The listing builds one solid part. Answer for the finished solid, in the listing's coordinates (mm). A direction names the side the tool comes from. Coordinates: 2 decimals unless noted, no trailing zeros. Order: outer loops, then holes, each group sorted by start corner. A loop starts at its lowest first (then second) coordinate and runs counter-clockwise, first axis right, second up. Notation, with made-up numbers: (20.25, 65.5) - (33.25, 65.5) arc R18 cw to (33.25, 78.5) - close; hole circle Ø7 at (-17.75, 75.25). An arc over 180 degrees is marked (long way). Use one line per item in the form item = value. Start each with the question number.
Item 1: Consider line 1 along Z through (x, y) = (6, -16.25); line 2 along Y through (x, z) = (9.25, 48.75); line 3 along X through (y, z) = (-17.5, 45.25). Determine where each line is inside the solid, lowest interval first. Write a range as [from, to].
Item 2: Section D-D, the plane x = 11.5 is taken. Write down the section's boundary in (y, z), and give its area (3 significant figures).
Item 3: A tool of negligible diameter and unlimited length cuts with its end or side. For faces 1 (the flat face through (10, -20, 46)), 2 (the flat face through (8, -15, 42.675)), from which of +Z, -Z, +X, -X, +Y, -Y can it reach the whole face along a straight path? Write none if from no direction.
Item 4: Section B-B, the plane x = 12.5 is taken. Write down the section's boundary in (y, z).
Item 5: Section A-A, the plane y = -3 is taken. Write down the section's boundary in (x, z).
Item 6: This flat-tipped pin is pushed along its axis until it touches: pin 1 Ø2 at (y, z) = (-16, 48) entering from -X. Where does it stop, or does it pass through?
Item 7: Section C-C, the plane z = 43.75 is taken. Write down the section's boundary in (x, y), and give its area (3 significant figures).
Item 8: The mould has two halves that part along Z. Classify faces 3 (the cylindrical face through (9.897, -3.57, 47.986)), 4 (the flat face through (10, 0, 46)), 5 (the flat face through (10, -10, 51.175)): released by +Z, released by -Z, zero draft, split by the parting line, or undercut.
from build123d import *

# Parameters (mm, degrees)
SKETCH1_W                 = 10
SKETCH1_H                 = 10
BOSS_EXTRUDE1_DEPTH       = 20
F_6_CLEARANCE_HOLE1_D     = 3.7973
F_6_CLEARANCE_HOLE1_DEPTH = 17
F_6_CLEARANCE_HOLE1_TIP   = 1.140824014
SKETCH2_W                 = 7
SKETCH2_H                 = 7
CUT_EXTRUDE1_DEPTH        = 7


with BuildPart() as part:
    # Sketch1 → Boss-Extrude1 (new body)
    with BuildSketch(Plane(origin=(0, 0, 0), x_dir=(1, 0, 0), z_dir=(0, 1, 0))):
        with Locations((9.826837964, -46.174693154)):
            Rectangle(SKETCH1_W, SKETCH1_H)
    extrude(amount=-BOSS_EXTRUDE1_DEPTH)

    # #6 Clearance Hole1
    with Locations(Plane(origin=(4.826837964, -3, 46.174693154), x_dir=(0, 0, -1), z_dir=(-1, 0, 0))):
        with Locations((0, 0)):
            Hole(F_6_CLEARANCE_HOLE1_D / 2, depth=F_6_CLEARANCE_HOLE1_DEPTH)
            with Locations((0, 0, -(F_6_CLEARANCE_HOLE1_DEPTH + F_6_CLEARANCE_HOLE1_TIP / 2))):  # 118° drill point
                Cone(0, F_6_CLEARANCE_HOLE1_D / 2, F_6_CLEARANCE_HOLE1_TIP, mode=Mode.SUBTRACT)

    # Sketch2 → Cut-Extrude1 (cut)
    with BuildSketch(Plane.ZY.offset(-4.826837964)):
        with Locations((46.174693154, -14.5)):
            Rectangle(SKETCH2_W, SKETCH2_H)
    extrude(amount=-CUT_EXTRUDE1_DEPTH, mode=Mode.SUBTRACT)


solid = part.part
Response:
q1.line_1 = [41.17, 42.67], [49.67, 51.17]
q1.line_2 = [-20, -18], [-11, 0]
q1.line_3 = [11.83, 14.83]
q2.outline = (-20, 41.17) - (0, 41.17) - (0, 51.17) - (-20, 51.17) - close; hole (-18, 42.67) - (-11, 42.67) - (-11, 49.67) - (-18, 49.67) - close; hole circle Ø3.8 at (-3, 46.17)
q2.area = 140 mm2
q3.face_1 = +Z, -Z, +X, -X, -Y
q3.face_2 = -X
q4.outline = (-20, 41.17) - (0, 41.17) - (0, 51.17) - (-20, 51.17) - close; hole circle Ø3.8 at (-3, 46.17)
q5.outline = (4.83, 41.17) - (14.83, 41.17) - (14.83, 44.28) - (4.83, 44.28) - close; (4.83, 48.07) - (14.83, 48.07) - (14.83, 51.17) - (4.83, 51.17) - close
q6.pin_1 = 11.83
q7.outline = (4.83, -20) - (14.83, -20) - (14.83, 0) - (4.83, 0) - (4.83, -11) - (11.83, -11) - (11.83, -18) - (4.83, -18) - close
q7.area = 151 mm2
q8.face_3 = undercut
q8.face_4 = zero draft
q8.face_5 = released by +Z
